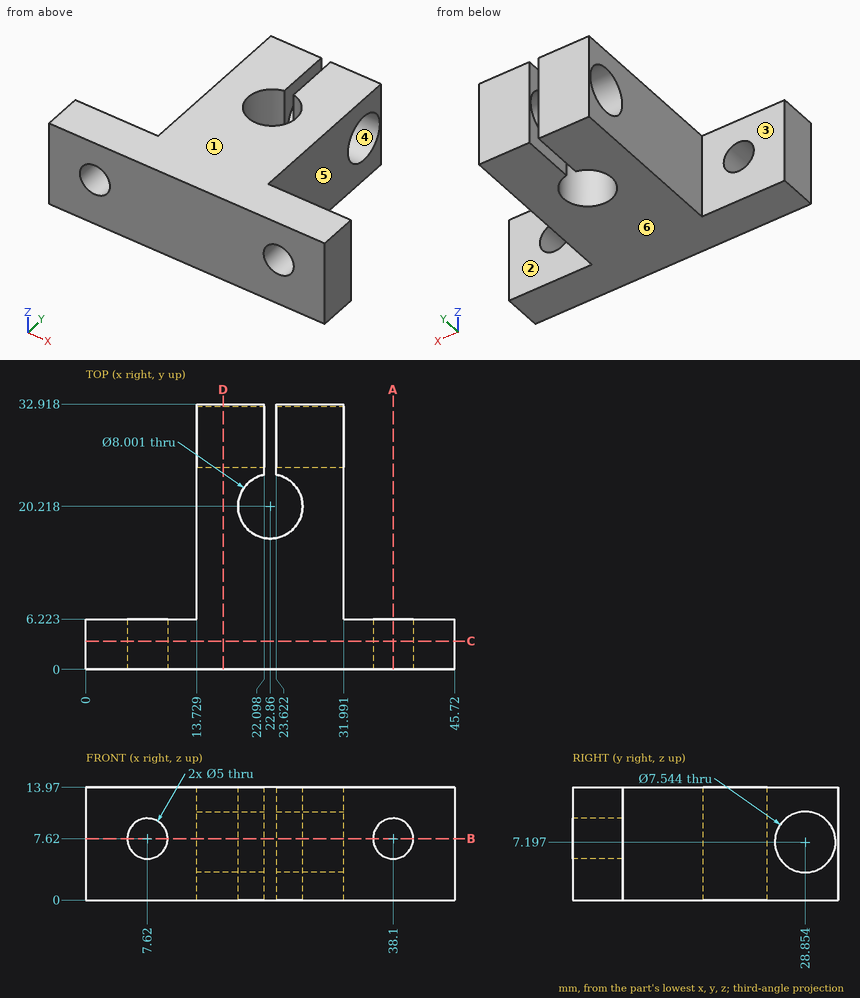
Source: three-view drawing plus pictorial views. Frame: mm from the lowest corner of the part. A direction names the side the tool comes from. Give positions to 0.01 mm unless a question says otherwise; leave off trailing zeros. Write each loop counter-clockwise with the first axis right and the second up, starting at its lowest first coordinate (ties: lowest second). Pieces come first, ordered by that corner, then holes. Notation, with made-up numbers: M -36.75,-8.5 L -5.75,-8.5 A26 ccw -5.75,11.5 Z; hole C -19,68 d9. An arc over 180 degrees is marked long. Use one line per item in the form item = value.
1. Cut plane C-C on y = 3.5. Return loops of the section in (x, z).
Outcome:
outline = M 0,0 L 45.72,0 L 45.72,13.97 L 0,13.97 Z; hole C 7.62,7.62 d5; hole C 38.1,7.62 d5
2. First-contact query: P1, Ø4.5, axis at x = 7.62, z = 7.62, coming from the -Y side; P2, Ø4, axis at x = 6.5, z = 8.5, coming from the +Y side; P3, Ø3, axis at y = 15.5, z = 7, coming from the +X side; P4, Ø6, axis at y = 24, z = 8, coming from the -X side. Flat tips, straight axial feed; report the tip coordinate or a pass-through.
Outcome:
P1 = through
P2 = 6.22
P3 = 31.99
P4 = 13.73
3. Mould query, pull axis Z, two halves, no side actions, for the marked faces 4, 5 and 6. Classes: released by +Z, released by -Z, zero draft, split by the parting line, or undercut.
Outcome:
face_4 = undercut
face_5 = zero draft
face_6 = released by -Z
4. Ray query, L1, parallel to Z at x = 7.62, y = 3.25; L2, parallel to X at y = 20.5, z = 1.75; L3, parallel to X at y = 24.5, z = 5.25. Return the intervals inside material, ascending.
Outcome:
L1 = 0 to 5.12, 10.12 to 13.97
L2 = 13.73 to 18.87, 26.85 to 31.99
L3 = 13.73 to 22.1, 23.62 to 31.99
5. Cut plane B-B on z = 7.62. State how many separate pieces and enclosed holes the cut face has, and give its area (3 significant figures).
Outcome:
separate_pieces = 5
enclosed_holes = 0
area = 521 mm²
6. Cut plane A-A on x = 38.1. Return loops of the section in (y, z).
Outcome:
outline = M 0,0 L 6.22,0 L 6.22,5.12 L 0,5.12 Z; M 0,10.12 L 6.22,10.12 L 6.22,13.97 L 0,13.97 Z
7. Cut plane D-D on x = 17. Return loops of the section in (y, z) (1 decimal), and give its area (3 significant figures).
Outcome:
outline = M 0,0 L 32.9,0 L 32.9,14 L 0,14 Z; hole C 28.9,7.2 d7.5
area = 415 mm²
8. Reachability of the marked faces 1, 2 and 3 from +Z, -Z, +X, -X, +Y, -Y: full face, straight path, thin tool, end or side. Return the list, or none.
Outcome:
face_1 = +Z, +X, -X, +Y, -Y
face_2 = +Z, -Z, +X, +Y
face_3 = +Z, -Z, -X, +Y
